Here's the drawing with two shaded views (mm, measured from the low corner). I have some questions. A direction names the side the tool comes from. Round coordinates to 2 decimals unless told otherwise and drop trailing zeros. Write each loop counter-clockwise with the first axis right and the second up, starting at its lowest first coordinate (ties: lowest second). Pieces come first, ordered by that corner, then holes. Notation, with made-up numbers: M 29,-2.75 L 53,-2.75 A16 cw 53,23.25 Z; hole C 39.25,35.5 d4. An arc over 180 degrees is marked long. Write item = value, one per line. Start each with the question number.
(1) On a 3-axis mill with a long thin cutter (end or side, diameter ignored), from which of +Z, -Z, +X, -X, +Y, -Y can I reach the whole of each face in a straight line? I mean the marked faces 1 and 2. Say none if no direction works.
(2) Will these pins go through, and if not, where does the flat tip stop? pin 1 Ø1 at (x, z) = (2.5, 7) entering from +Y; pin 2 Ø1.5 at (x, y) = (1, 0.5) entering from -Z.
(3) I want a section at C-C (z = 5). List the corners of the cut face in (x, y) for me.
(4) I want a section at A-A (x = 2.4). List the corners of the cut face in (y, z) for me.
(5) I need wall thicknesses on line 1 along Y through (x, z) = (2.4, 4); line 2 along Z through (x, y) = (1.65, 4.3); line 3 along Y through (x, z) = (1.5, 6). Which ranges of each line are inside material? Lowest first, please.
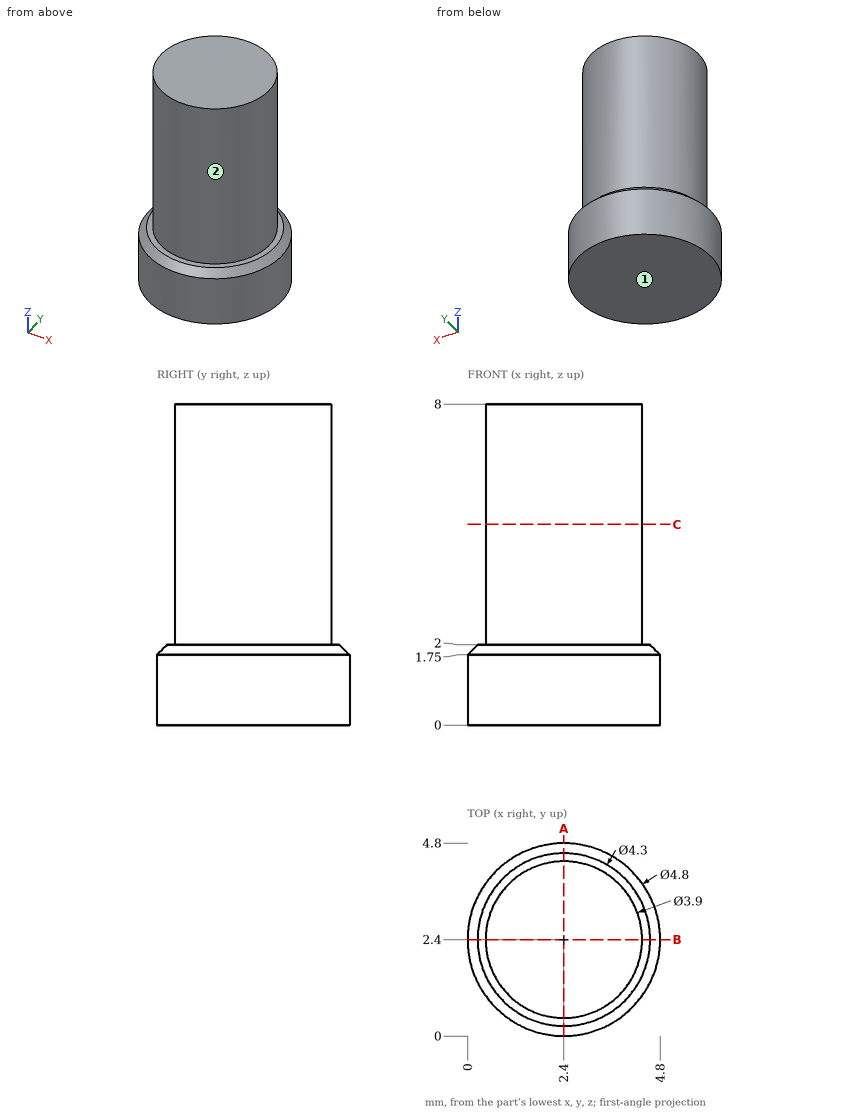
Returned:
q1.face_1 = -Z, +X, -X, +Y, -Y
q1.face_2 = +Z
q2.pin_1 = 4.35
q2.pin_2 = 0
q3.outline = C 2.4,2.4 d3.9
q4.outline = M 0,0 L 4.8,0 L 4.8,1.75 L 4.55,2 L 4.35,2 L 4.35,8 L 0.45,8 L 0.45,2 L 0.25,2 L 0,1.75 Z
q5.line_1 = 0.45 to 4.35
q5.line_2 = 0 to 2
q5.line_3 = 0.67 to 4.13
